from build123d import *

# Parameters (mm, degrees)
BOSS_EXTRUDE1_DEPTH = 80
SKETCH2_R           = 5.5
SKETCH2_R_2         = 3.9
BOSS_EXTRUDE2_DEPTH = 20
SKETCH3_R           = 6
BOSS_EXTRUDE3_DEPTH = 12
FILLET1_R           = 5
BOSS_EXTRUDE4_DEPTH = 4
FILLET2_R           = 1


with BuildPart() as part:
    # Sketch1 → Boss-Extrude1 (new body)
    with BuildSketch(Plane(origin=(0, 0, 0), x_dir=(1, 0, 0), z_dir=(0, 1, 0))):
        with BuildLine():
            Line((11.521718622, 12.5), (19.306734576, 12.5))
            ThreePointArc((19.306734576, 12.5), (23, 0), (19.306734576, -12.5))
            Line((19.306734576, -12.5), (11.521718622, -12.5))
            ThreePointArc((11.521718622, -12.5), (-17, 0), (11.521718622, 12.5))
        make_face()
    extrude(amount=BOSS_EXTRUDE1_DEPTH)

    # Sketch2 → Boss-Extrude2 (add)
    with BuildSketch(Plane(origin=(0, 80, 0), x_dir=(1, 0, 0), z_dir=(0, 1, 0))):
        with Locations(Location((17, 0, 0), (0, 0, 270))):
            Circle(SKETCH2_R)
        with Locations(Location((17, 0, 0), (0, 0, 270))):
            Circle(SKETCH2_R_2, mode=Mode.SUBTRACT)
    extrude(amount=BOSS_EXTRUDE2_DEPTH)

    # Sketch3 → Boss-Extrude3 (add)
    with BuildSketch(Plane(origin=(0, 80, 0), x_dir=(1, 0, 0), z_dir=(0, 1, 0))):
        with Locations(Location((-3, 0, 0), (0, 0, 270))):
            Circle(SKETCH3_R)
    extrude(amount=BOSS_EXTRUDE3_DEPTH)

    # Fillet1
    fillet1_edges = [part.edges().sort_by_distance(p)[0] for p in [
        (-3, 80, -6),
    ]]
    fillet(fillet1_edges, radius=FILLET1_R)

    # Sketch4 → Boss-Extrude4 (add)
    with BuildSketch(Plane.XZ):
        with BuildLine():
            Line((-7.116025404, 10.325317547), (-8.366025404, 12.490381057))
            ThreePointArc((-8.366025404, 12.490381057), (-8, 13.856406461), (-6.633974596, 13.490381057))
            Line((-6.633974596, 13.490381057), (-5.383974596, 11.325317547))
            ThreePointArc((-5.383974596, 11.325317547), (-5.75, 9.959292144), (-7.116025404, 10.325317547))
        make_face()
        with BuildLine():
            Line((-5.383974596, -11.325317547), (-6.633974596, -13.490381057))
            ThreePointArc((-6.633974596, -13.490381057), (-8, -13.856406461), (-8.366025404, -12.490381057))
            Line((-8.366025404, -12.490381057), (-7.116025404, -10.325317547))
            ThreePointArc((-7.116025404, -10.325317547), (-5.75, -9.959292144), (-5.383974596, -11.325317547))
        make_face()
        with BuildLine():
            Line((18.75, 1), (21.25, 1))
            ThreePointArc((21.25, 1), (22.25, 0), (21.25, -1))
            Line((21.25, -1), (18.75, -1))
            ThreePointArc((18.75, -1), (17.75, 0), (18.75, 1))
        make_face()
    extrude(amount=BOSS_EXTRUDE4_DEPTH)

    # Fillet2
    fillet2_edges = [part.edges().sort_by_distance(p)[0] for p in [
        (11.521718622, 40, -12.5),
        (19.306734576, 40, -12.5),
        (19.306734576, 40, 12.5),
        (11.521718622, 40, 12.5),
    ]]
    fillet(fillet2_edges, radius=FILLET2_R)


solid = part.part
Model file for the job. Use its own axes, mm. A direction names the side the tool comes from. Give positions to 0.01 mm unless a question says otherwise; leave off trailing zeros. Loops run counter-clockwise (first coordinate to the right, second up) from the corner with the lowest first, then second, coordinate; pieces in that order, holes last. Notation, with made-up numbers: (29, 51) -> (56, 51) arc R11 ccw to (56, 67) -> close; hole circle Ø4 at (89.25, -29.5). An arc over 180 degrees is marked (long way). Use a Markdown table: item, result. Add a question column.
(1) Tool access for faces 5 (the cylindrical face through (22.25, -1.97, 0.02)), 6 (the flat face through (20, -2, 1)), 7 (the cylindrical face through (-8.019, -1.972, 13.845)): list every direction of +Z, -Z, +X, -X, +Y, -Y with a clear straight run to the whole face (end or side of a thin tool).
(2) Drop flat-ended pins along their axis: pin 1 Ø2 at (x, y) = (5.5, 79.5) entering from +Z; pin 2 Ø6 at (x, z) = (-10, -8.5) entering from +Y; pin 3 Ø12 at (x, y) = (18, 56) entering from -Z. Give the stop position or say it passes through.
(3) Slice it at C-C on x = 15. List the corners of the cut face in (y, z).
(4) Slice it at A-A on z = 0. List the corners of the cut face in (x, y), and give its area (3 significant figures).
(5) Mould opens along Z. For faces 1 (the cylindrical face through (-5.73, -1.97, 9.97)), 2 (the cylindrical face through (-1.198, 88.451, 5.723)), 3 (the flat face through (20, -4, 0)), 4 (the cylindrical face through (-5.77, -1.97, -9.95)) say: +Z half, -Z half, draft (parallel to the pull), parting line (faces both ways), or undercut.
(6) Wall check: line 1 along X through (y, z) = (88, 0); line 2 along X through (y, z) = (94, 0); line 3 along Y through (x, z) = (-3, -12). Give the ranges that are in metal, low to high.
Filled sheet:
| question | item | result |
|---|---|---|
| 1 | face 5 | +X, -Y |
| 1 | face 6 | +Z, +X, -X, -Y |
| 1 | face 7 | -Y |
| 2 | pin 1 | z = 16.39 |
| 2 | pin 2 | y = 80.99 |
| 2 | pin 3 | z = -12.5 |
| 3 | outline | (0, -12.5) -> (80, -12.5) -> (80, -5.12) -> (100, -5.12) -> (100, -3.35) -> (80, -3.35) -> (80, 3.35) -> (100, 3.35) -> (100, 5.12) -> (80, 5.12) -> (80, 12.5) -> (0, 12.5) -> close |
| 4 | outline | (-17, 0) -> (17.75, 0) -> (17.75, -4) -> (22.25, -4) -> (22.25, 0) -> (23, 0) -> (23, 80) -> (22.5, 80) -> (22.5, 100) -> (20.9, 100) -> (20.9, 80) -> (13.1, 80) -> (13.1, 100) -> (11.5, 100) -> (11.5, 80) -> (8, 80) arc R5 cw to (3, 85) -> (3, 92) -> (-9, 92) -> (-9, 85) arc R5 cw to (-14, 80) -> (-17, 80) -> close |
| 4 | area | 3,440 mm2 |
| 5 | face 1 | undercut |
| 5 | face 2 | parting line |
| 5 | face 3 | draft |
| 5 | face 4 | undercut |
| 6 | line 1 | -9 to 3, 11.5 to 13.1, 20.9 to 22.5 |
| 6 | line 2 | 11.5 to 13.1, 20.9 to 22.5 |
| 6 | line 3 | 0 to 80 |
